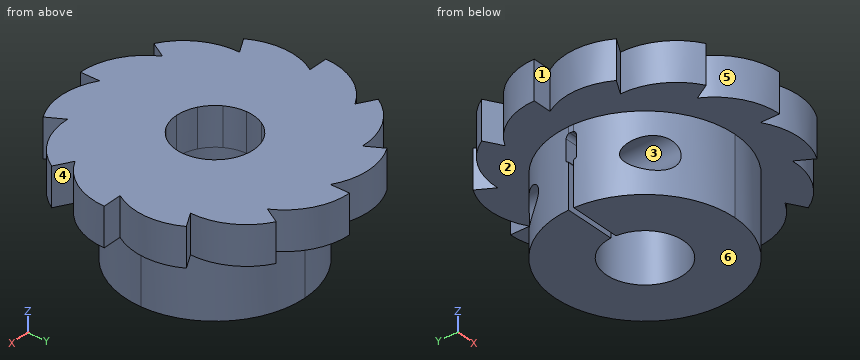
from build123d import *
from build123d.topology import SkipClean

# Parameters (mm, degrees)
BOSS_EXTRUDE1_DEPTH = 3
CIRPATTERN1_COUNT   = 12
BOSS_EXTRUDE2_START = 6
SKETCH3_R           = 3
BOSS_EXTRUDE2_DEPTH = 6
SKETCH4_R           = 1.25
CUT_EXTRUDE1_DEPTH  = 22.272047386
CUT_EXTRUDE3_REACH  = 23.272
FILLET2_R           = 0.1
FILLET3_R           = 0.3
CUT_EXTRUDE4_DEPTH  = 6


with BuildPart() as part:
    # Sketch1 → Boss-Extrude1 (new body)
    with BuildSketch(Plane.XY):
        with BuildLine():
            Line((0, 9), (0, 10.5))
            ThreePointArc((0, 10.5), (2.62541419, 9.771470047), (4.5, 7.794228634))
            Line((4.5, 7.794228634), (1.5, 2.598076211))
            ThreePointArc((1.5, 2.598076211), (0.776457135, 2.897777479), (0, 3))
            Line((0, 3), (0, 9))
        make_face()
    boss_extrude1 = extrude(amount=BOSS_EXTRUDE1_DEPTH)

    # CirPattern1: Boss-Extrude1 ×12 about axis
    cirpattern1_axis = Axis((0, 0, 0), (0, 0, 1))
    for i in range(1, CIRPATTERN1_COUNT):
        add(boss_extrude1.rotate(cirpattern1_axis, i * 360 / CIRPATTERN1_COUNT))

    # Sketch3 → Boss-Extrude2 (add)
    with SkipClean():  # the faces are left unmerged after this step: merging them gives an invalid solid
        with BuildSketch(Plane(origin=(0, 0, 0), x_dir=(-1, 0, 0), z_dir=(0, 0, -1)).offset(BOSS_EXTRUDE2_START)):
            with BuildLine():
                Line((7, 0), (7, -7))
                Line((7, -7), (0, -7))
                ThreePointArc((0, -7), (-4.949747468, -4.949747468), (-7, 0))
                Line((-7, 0), (-7, 7))
                Line((-7, 7), (7, 7))
                Line((7, 7), (7, 0))
            make_face()
            Circle(SKETCH3_R, mode=Mode.SUBTRACT)
        extrude(amount=-BOSS_EXTRUDE2_DEPTH)

    # Sketch4 → Cut-Extrude1 (cut, through all)
    with SkipClean():  # the faces are left unmerged after this step: merging them gives an invalid solid
        with BuildSketch(Plane(origin=(0, 7, 0), x_dir=(1, 0, 0), z_dir=(0, 1, 0))):
            with Locations(Location((-5, 3, 0), (0, 0, 270))):
                Circle(SKETCH4_R)
        extrude(amount=-CUT_EXTRUDE1_DEPTH, mode=Mode.SUBTRACT)

    # Sketch6 → Cut-Extrude3 (cut, up to next)
    with BuildSketch(Plane.ZY.offset(7), mode=Mode.PRIVATE) as cut_extrude3_sk1:
        Polygon((-6, -0.2), (-6, 0.2), (-2.5, 0.2), (-2.5, 0.4), (-0.5, 0.4), (-0.5, -0.4), (-2.5, -0.4), (-2.5, -0.2), align=None)
    cut_extrude3_tool1 = extrude(cut_extrude3_sk1.sketch, amount=-CUT_EXTRUDE3_REACH, mode=Mode.PRIVATE) & part.part
    add(cut_extrude3_tool1.solids().sort_by_distance((-7, 0, -2.783333))[0], mode=Mode.SUBTRACT)

    # Fillet2
    fillet2_edges = [part.edges().sort_by_distance(p)[0] for p in [
        (-6.572821962, 0.4, -2.5),
        (-3.423840993, 0.2, -2.5),
        (-3.413784913, 0.4, -2.5),
        (-6.572821962, 0.2, -2.5),
        (-3.413784913, -0.4, -2.5),
        (-3.423840993, -0.2, -2.5),
        (-6.572821962, -0.4, -2.5),
        (-6.572821962, -0.2, -2.5),
    ]]
    fillet(fillet2_edges, radius=FILLET2_R - 0.0001)  # a hair under: the kernel refuses the full size

    # Fillet3
    fillet3_edges = [part.edges().sort_by_distance(p)[0] for p in [
        (-4.986606875, 0.4, -0.5),
        (-4.986606875, -0.4, -0.5),
    ]]
    fillet(fillet3_edges, radius=FILLET3_R)

    # Sketch7 → Cut-Extrude4 (cut)
    with SkipClean():  # the faces are left unmerged after this step: merging them gives an invalid solid
        with BuildSketch(Plane(origin=(0, 0, -6), x_dir=(-1, 0, 0), z_dir=(0, 0, -1))):
            with BuildLine():
                Line((0, 7), (-7, 7))
                Line((-7, 7), (-7, 0))
                ThreePointArc((-7, 0), (-4.949747468, 4.949747468), (0, 7))
            make_face()
            with BuildLine():
                Line((7, 7), (0, 7))
                ThreePointArc((0, 7), (4.878524367, 5.019960159), (6.997142274, 0.2))
                Line((6.997142274, 0.2), (7, 0.2))
                Line((7, 0.2), (7, 7))
            make_face()
            with BuildLine():
                Line((7, -7), (7, -0.2))
                Line((7, -0.2), (6.997142274, -0.2))
                ThreePointArc((6.997142274, -0.2), (4.878524367, -5.019960159), (0, -7))
                Line((0, -7), (7, -7))
            make_face()
        extrude(amount=-CUT_EXTRUDE4_DEPTH, mode=Mode.SUBTRACT)


solid = part.part
Build history of the part. All positions in model axes, mm. Face numbers are marked on the shaded views. A direction names the side the tool comes from. Coordinates: 2 decimals unless noted, no trailing zeros. Write each loop counter-clockwise with the first axis right and the second up, starting at its lowest first coordinate (ties: lowest second). Pieces come first, ordered by that corner, then holes.
(1) Mould opens along X. For the marked faces 4, 5 and 6 say: pulls with the +X half, pulls with the -X half, needs draft (parallel to the pull), parting line crosses it, or undercut.
(2) Cut at A-A on z = -2. List the corners of the cut face in (x, y).
(3) Cut at B-B on y = -8.75. List the corners of the cut face in (x, z).
(4) 3-axis set-ups, long thin cutter, end or side, ignore diameter. For the marked faces 1, 2 and 3: which of +Z, -Z, +X, -X, +Y, -Y reach the whole face in a straight line?
(5) Cut at C-C on x = -5. List the corners of the cut face in (y, z), and give its area (3 significant figures).
(6) Drill centre lines: line 1 (Z direction, x = -5, y = 2.55); line 2 (X direction, y = 2.25, z = -4); line 3 (Z direction, x = -4, y = 6.5). Where is each one in solid material? Low to high.
(7) Pin check, flat tips, straight feed: pin 1 Ø0.5 at (x, z) = (-9.5, 1) entering from -Y; pin 2 Ø1 at (x, z) = (3.5, 2) entering from +Y; pin 3 Ø2 at (y, z) = (-1, -4) entering from -X; pin 4 Ø5.5 at (x, y) = (0, 0) entering from -Z. Stop position of each tip, or through.
(8) Cut at D-D on y = -5.5. List the corners of the cut face in (x, z).
Working result:
1. face 4: pulls with the +X half
1. face 5: undercut
1. face 6: needs draft
2. outline: (-6.99, -0.4) arc R7 ccw to (-5.75, -3.99) - (-5.75, -0.4) - close; (-6.99, 0.4) - (-5.75, 0.4) - (-5.75, 3.99) arc R7 ccw to start; (-4.25, -5.56) arc R7 ccw (long way) to (-4.25, 5.56) - (-4.25, 0.4) - (-2.97, 0.4) arc R3 cw (long way) to (-2.97, -0.4) - (-4.25, -0.4) - close
3. outline: (-5.77, 0) - (-5.05, 0) - (-5.05, 3) - (-5.77, 3) - close; (-3.84, 0) - (5.05, 0) - (5.05, 3) - (-3.84, 3) - close
4. face 1: +Z, -Z, -X
4. face 2: -Z
4. face 3: +Y, -Y
5. outline: (-8.66, 0) - (-4.9, 0) - (-4.9, -1.75) - (-0.4, -1.75) - (-0.4, -0.8) arc R0.3 cw to (-0.1, -0.5) - (0.1, -0.5) arc R0.3 cw to (0.4, -0.8) - (0.4, -1.75) - (4.9, -1.75) - (4.9, 0) - (7.79, 0) - (7.79, 3) - (-8.66, 3) - close; (-4.9, -6) - (-0.2, -6) - (-0.2, -4.25) - (-4.9, -4.25) - close; (0.2, -6) - (4.9, -6) - (4.9, -4.25) - (0.2, -4.25) - close; (8.66, 0) - (9.23, 0) - (9.23, 3) - (8.66, 3) - close
5. area: 83.7 mm2
6. line 1: z = -6 to -4.25, -1.75 to 3
6. line 2: x = -6.63 to -5.75, -4.25 to -1.98, 1.98 to 6.63
6. line 3: z = 0 to 3
7. pin 1: stops at y = -4.96
7. pin 2: stops at y = 9.52
7. pin 3: stops at x = -7
7. pin 4: passes through
8. outline: (-7.73, 0) - (-4.33, 0) - (-4.33, -1.94) arc R1.25 cw to (-4.33, -4.06) - (-4.33, -6) - (4.33, -6) - (4.33, 0) - (8.94, 0) - (8.94, 3) - (-7.73, 3) - close
